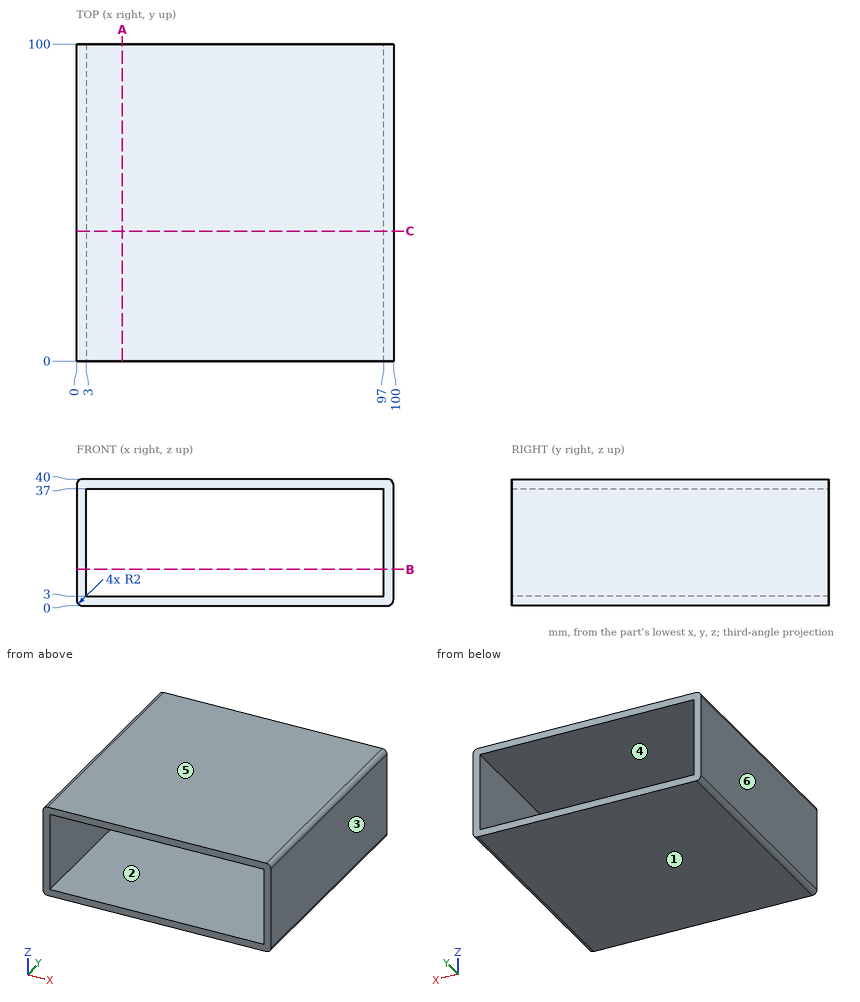
Print and shaded views of the part. All mm, measured from the part's lowest x, y and z. A direction names the side the tool comes from. Give positions to 0.01 mm unless a question says otherwise; leave off trailing zeros. Loops run counter-clockwise (first coordinate to the right, second up) from the corner with the lowest first, then second, coordinate; pieces in that order, holes last.
1) Pull direction X, two halves, no side cores. Call the marked faces 3, 4, 5 and 6: +X half, -X half, draft (parallel to the pull), parting line (faces both ways), or undercut.
2) Wall check: line 1 (X direction, y = 49, z = 3.5); line 2 (Z direction, x = 49.5, y = 4.5). Give the ranges that are in metal, low to high.
3) Saw through at C-C (y = 41). Write the cut outline in (x, z).
4) Tool access for the marked faces 1 and 2: list every direction of +Z, -Z, +X, -X, +Y, -Y with a clear straight run to the whole face (end or side of a thin tool).
5) Saw through at B-B (z = 11.5). Write the cut outline in (x, y), plus the area to 3 significant figures.
6) Flat gauge pin, fed straight in: pin 1 Ø12 at (x, z) = (29.5, 6) entering from -Y. Where does the tip first touch, or does it go through?
7) Saw through at A-A (x = 14.5). Write the cut outline in (y, z), plus the area to 3 significant figures.
Answer block:
1. face 3: +X half
1. face 4: undercut
1. face 5: draft
1. face 6: -X half
2. line 1: x = 0 to 3, 97 to 100
2. line 2: z = 0 to 3, 37 to 40
3. outline: (0, 2) arc R2 ccw to (2, 0) - (98, 0) arc R2 ccw to (100, 2) - (100, 38) arc R2 ccw to (98, 40) - (2, 40) arc R2 ccw to (0, 38) - close; hole (3, 3) - (97, 3) - (97, 37) - (3, 37) - close
4. face 1: -Z, +X, -X, +Y, -Y
4. face 2: +Y, -Y
5. outline: (0, 0) - (3, 0) - (3, 100) - (0, 100) - close; (97, 0) - (100, 0) - (100, 100) - (97, 100) - close
5. area: 600 mm2
6. pin 1: stops at y = 0
7. outline: (0, 0) - (100, 0) - (100, 3) - (0, 3) - close; (0, 37) - (100, 37) - (100, 40) - (0, 40) - close
7. area: 600 mm2
